Autodesk Inventor part; units mm, degrees
ref_plane "WorkPlane1" through (0, 0, 0) normal (0, 0, 1) x (1, 0, 0)
ref_plane "MSC_PF1" through (0, 0, 0) normal (1, 0, 0) x (0, 1, 0)
ref_plane "MSC_PT1" through (0, 0, 0) normal (0, 0, -1) x (-1, 0, 0)
ref_plane "WorkPlane1" through (0, 0, 0) normal (0, 0, 1) x (1, 0, 0)
sketch "Sketch1" plane through (0, 0, 0) normal (0, 0, 1) x (1, 0, 0)
  point P0 (0, 0)
sketch "Sketch2" plane through (0, 0, 0) normal (0, 0, 1) x (1, 0, 0)
  line L0 (-6.5, 3.7529) -> (-6.5, -3.7529)
  line L1 (0, 7.5054) -> (-6.5, 3.7529)
  line L2 (6.5, 3.7529) -> (0, 7.5054)
  line L3 (6.5, -3.7529) -> (6.5, 3.7529)
  line L4 (0, -7.5054) -> (6.5, -3.7529)
  line L5 (-6.5, -3.7529) -> (0, -7.5054)
  circle A0 centre (0, 0) radius 6.5 construction
  dimension "d1" = 13
  dimension "d29" = 0
  dimension "d30" = 0
extrude "Extrusion1" add sketch "Sketch2" along normal blind 5.3
sketch "Sketch3" plane through (0, 0, 0) normal (1, 0, 0) x (0, 1, 0)
  line L0 (6.5, 5.3) -> (7.6054, 5.3)
  line L1 (7.6054, 4.6618) -> (6.5, 5.3)
  line L2 (7.6054, 5.3) -> (7.6054, 4.6618)
  line L3 (0, -1.06) -> (0, 6.36)
  line L4 (7.5054, 0) -> (7.5054, 5.3)
  dimension "d25" = 0.1
  dimension "d26" = 0
  dimension "d27" = 60
  dimension "d28" = 6.5
revolve "Revolution1" cut sketch "Sketch3" angle 360 about axis through (0, 0, -10) along (0, 0, 1)
sketch "Sketch4" plane through (0, 0, 0) normal (1, 0, 0) x (0, 1, 0)
  line L0 (0, -45) -> (0, 0)
  line L1 (-4, -45) -> (0, -45)
  line L2 (-4, 0) -> (-4, -45)
  line L3 (0, 0) -> (-4, 0)
  line L4 (0, -45) -> (0, 0)
  line L5 (-4.8, 0) -> (0.8, 0)
  line L6 (0, -54) -> (0, 9)
  dimension "d18" = 4
  dimension "d20" = 45
  dimension "d33" = 0
  dimension "d34" = 0
revolve "Revolution2" add sketch "Sketch4" angle 360 about axis through (0, 0, -45) along (0, 0, -1)
chamfer "Chamfer1" distance 0.625 angle 45 1 edges at (0, 4, -45)
fillet "Fillet1" radius 0.4 1 edges at (0, 4, 0)
thread "Thread1"
ref_plane "MSC_PF1" through (0, 0, 0) normal (1, 0, 0) x (0, 1, 0)
ref_plane "MSC_PT1" through (0, 0, 0) normal (0, 0, -1) x (-1, 0, 0)
equation "\"d22\" = 0.5 * PTC"
equation "\"d23\" = 0.5 * PTC"
equation "\"d24\" = r"
equation "\"d1\" = ParS"
equation "\"d6\" = ParK"
equation "\"b\" = NLG - 2 * PTC"
equation "\"d28\" = 0.5 * ParS"
equation "\"d18\" = 0.5 * NND"
equation "\"d20\" = NLG"
equation "\"NND\" = 8"
equation "\"NLG\" = 45"
equation "\"PTC\" = 1.25"
equation "\"ParK\" = 5.3"
equation "\"ParS\" = 13"
equation "\"msp_es\" = 0.577367 * ParS"
equation "\"r\" = 0.4"
equation "\"THREADDIA\" = NND"
properties part number "ISO 4018 - M8 x 45" material "Steel"
Check sheet for the modelled part. Datum: model origin and axes. Units: mm. A direction names the side the tool comes from. Round coordinates to 2 decimals unless told otherwise and drop trailing zeros. Order: outer loops, then holes, each group sorted by start corner. A loop starts at its lowest first (then second) coordinate and runs counter-clockwise, first axis right, second up.
1) Tool access check on faces 1 (the flat face through (-4.4, -1.6, 0)), 2 (the conical face through (0.02, -6.71, 5.18)). Record the directions out of +Z, -Z, +X, -X, +Y, -Y that give a thin tool (end or side, any length) a straight path to the whole face; none if there is none.
2) Go/stop test with flat-tipped pins: pin 1 Ø1.5 at (x, y) = (-5, -3.5) entering from -Z; pin 2 Ø4 at (x, z) = (0.5, -36) entering from -Y; pin 3 Ø3 at (x, z) = (3.5, -19.5) entering from -Y. Record where each tip stops, or that it passes through.
3) Scan lines: line 1 (Z direction, x = -0.5, y = 5); line 2 (X direction, y = -4.25, z = 1); line 3 (Z direction, x = 3.5, y = -0.5). Record each from-to range of solid material in increasing order.
4) Section check A-A (z = -14). Record the boundary of the cut face in (x, y), and give its area (3 significant figures).
Result:
1. face 1: -Z
1. face 2: +Z, -Y
2. pin 1: stops at z = 0
2. pin 2: stops at y = -4
2. pin 3: stops at y = -3.46
3. line 1: z = 0 to 5.3
3. line 2: x = -5.64 to 5.64
3. line 3: z = -44.84 to 5.3
4. outline: circle Ø8 at (0, 0)
4. area: 50.3 mm2
